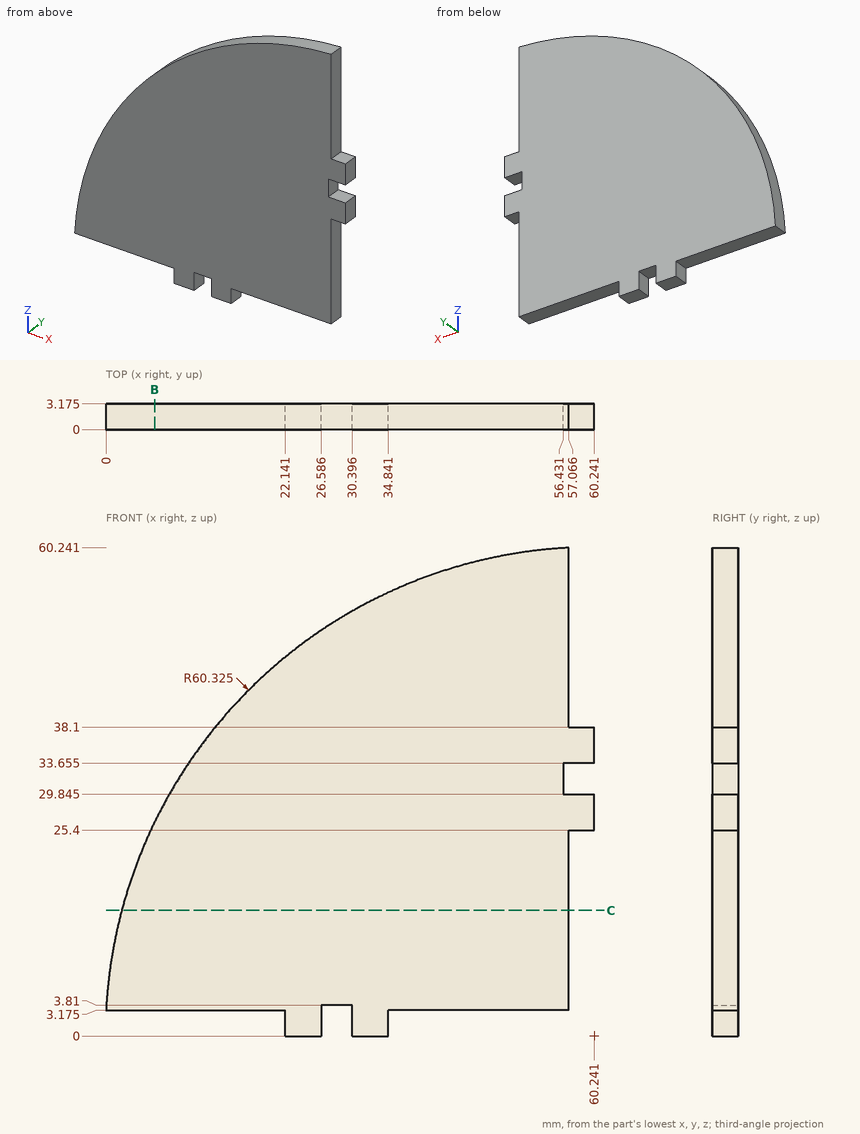
Answer from the drawing. Dimensions are ordinates in mm from the lowest x, y and z of the part. Round coordinates to 2 decimals unless told otherwise and drop trailing zeros. Loops run counter-clockwise (first coordinate to the right, second up) from the corner with the lowest first, then second, coordinate; pieces in that order, holes last. Notation, with made-up numbers: (39.5, -17) - (60.5, -17) arc R15 cw to (60.5, -6) - close; hole circle Ø3 at (-14, 71.25). An arc over 180 degrees is marked (long way). Return JSON: item names as keys, results as strings. Group by question number.
1. The part is cut by section B-B on x = 6. Determine the outline of the cut face in (y, z) (1 decimal).
2. Each of these flat-tipped pins is pushed along its axis until it touches: P1, Ø1.5, axis at y = 1, z = 8, coming from the +X side; P2, Ø1.6, axis at x = 59.5, y = 1.5, coming from the -Z side; P3, Ø1, axis at y = 1, z = 2, coming from the +X side. Where does it stop, or does it pass through?
3. Consider probe 1 along Z at (x, y) = (56.5, 1.15) (1 decimal); probe 2 along Z at (x, y) = (34, 0.45); probe 3 along Z at (x, y) = (52, 2.05) (1 decimal). Determine where each line is inside the solid, lowest interval first.
4. The part is cut by section C-C on z = 15.5. Determine the outline of the cut face in (x, y) (1 decimal), then the cut area to 3 significant figures.
Resolved:
{
 "1": {"outline": "(0, 3.2) - (3.2, 3.2) - (3.2, 26.4) - (0, 26.4) - close"},
 "2": {"P1": "stops at x = 57.07", "P2": "stops at z = 25.4", "P3": "stops at x = 34.84"},
 "3": {"probe 1": "z = 3.2 to 29.8, 33.7 to 60.2", "probe 2": "z = 0 to 54.32", "probe 3": "z = 3.2 to 59.8"},
 "4": {"outline": "(1.9, 0) - (57.1, 0) - (57.1, 3.2) - (1.9, 3.2) - close", "area": "175 mm²"}
}
